```python
from build123d import *

# Parameters (mm, degrees)
BOSS_EXTRUDE1_DEPTH  = 4
MIRROR6_COPY_1_DEPTH = 4
MIRROR6_COPY_2_DEPTH = 4


with BuildPart() as part:
    # Sketch1 → Boss-Extrude1 (new body)
    with BuildSketch(Plane(origin=(0, 0, 0), x_dir=(1, 0, 0), z_dir=(0, 1, 0))):
        with BuildLine():
            Line((-290, 108.284271247), (-290, 0))
            Line((-290, 0), (-205.5, 0))
            ThreePointArc((-205.5, 0), (-202.131727984, 8.131727984), (-194, 11.5))
            Line((-194, 11.5), (-186, 11.5))
            ThreePointArc((-186, 11.5), (-177.868272016, 8.131727984), (-174.5, 0))
            Line((-174.5, 0), (0, 0))
            Line((0, 0), (0, 40))
            Line((0, 40), (-221.715728753, 40))
            Line((-221.715728753, 40), (-250, 68.284271247))
            Line((-250, 68.284271247), (-250, 108.284271247))
            Line((-250, 108.284271247), (-290, 108.284271247))
        make_face()
        with BuildLine():
            ThreePointArc((-207.499780644, 13.499780644), (-209.499780644, 15.499780644), (-207.499780644, 17.499780644))
            Line((-207.499780644, 17.499780644), (-203.499780644, 17.499780644))
            ThreePointArc((-203.499780644, 17.499780644), (-201.499780644, 15.499780644), (-203.499780644, 13.499780644))
            Line((-203.499780644, 13.499780644), (-207.499780644, 13.499780644))
        make_face(mode=Mode.SUBTRACT)
        with BuildLine():
            Line((-176.500219356, 17.499780644), (-172.500219356, 17.499780644))
            ThreePointArc((-172.500219356, 17.499780644), (-170.500219356, 15.499780644), (-172.500219356, 13.499780644))
            Line((-172.500219356, 13.499780644), (-176.500219356, 13.499780644))
            ThreePointArc((-176.500219356, 13.499780644), (-178.500219356, 15.499780644), (-176.500219356, 17.499780644))
        make_face(mode=Mode.SUBTRACT)
    boss_extrude1 = extrude(amount=BOSS_EXTRUDE1_DEPTH)

    # Mirror1: Boss-Extrude1 across plane
    add(boss_extrude1.mirror(Plane(origin=(0, 4, 0), x_dir=(1, 0, 0), z_dir=(0, 0, -1))))

    # Mirror5: Boss-Extrude1 across plane
    add(boss_extrude1.mirror(Plane(origin=(0, 4, 0), x_dir=(0, 0, 1), z_dir=(1, 0, 0))))

    # Mirror6 copy 1 sketch → Mirror6 copy 1 (add)
    with BuildSketch(Plane(origin=(0, 0, 0), x_dir=(-1, 0, 0), z_dir=(0, 1, 0))):
        with BuildLine():
            Line((-290, 108.284271247), (-290, 0))
            Line((-290, 0), (-205.5, 0))
            ThreePointArc((-205.5, 0), (-202.131727984, 8.131727984), (-194, 11.5))
            Line((-194, 11.5), (-186, 11.5))
            ThreePointArc((-186, 11.5), (-177.868272016, 8.131727984), (-174.5, 0))
            Line((-174.5, 0), (0, 0))
            Line((0, 0), (0, 40))
            Line((0, 40), (-221.715728753, 40))
            Line((-221.715728753, 40), (-250, 68.284271247))
            Line((-250, 68.284271247), (-250, 108.284271247))
            Line((-250, 108.284271247), (-290, 108.284271247))
        make_face()
        with BuildLine():
            ThreePointArc((-207.499780644, 13.499780644), (-209.499780644, 15.499780644), (-207.499780644, 17.499780644))
            Line((-207.499780644, 17.499780644), (-203.499780644, 17.499780644))
            ThreePointArc((-203.499780644, 17.499780644), (-201.499780644, 15.499780644), (-203.499780644, 13.499780644))
            Line((-203.499780644, 13.499780644), (-207.499780644, 13.499780644))
        make_face(mode=Mode.SUBTRACT)
        with BuildLine():
            Line((-176.500219356, 17.499780644), (-172.500219356, 17.499780644))
            ThreePointArc((-172.500219356, 17.499780644), (-170.500219356, 15.499780644), (-172.500219356, 13.499780644))
            Line((-172.500219356, 13.499780644), (-176.500219356, 13.499780644))
            ThreePointArc((-176.500219356, 13.499780644), (-178.500219356, 15.499780644), (-176.500219356, 17.499780644))
        make_face(mode=Mode.SUBTRACT)
    extrude(amount=MIRROR6_COPY_1_DEPTH)

    # Mirror6 copy 2 sketch → Mirror6 copy 2 (add)
    with BuildSketch(Plane(origin=(0, 0, 0), x_dir=(1, 0, 0), z_dir=(0, 1, 0))):
        with BuildLine():
            Line((-290, -108.284271247), (-290, 0))
            Line((-290, 0), (-205.5, 0))
            ThreePointArc((-205.5, 0), (-202.131727984, -8.131727984), (-194, -11.5))
            Line((-194, -11.5), (-186, -11.5))
            ThreePointArc((-186, -11.5), (-177.868272016, -8.131727984), (-174.5, 0))
            Line((-174.5, 0), (0, 0))
            Line((0, 0), (0, -40))
            Line((0, -40), (-221.715728753, -40))
            Line((-221.715728753, -40), (-250, -68.284271247))
            Line((-250, -68.284271247), (-250, -108.284271247))
            Line((-250, -108.284271247), (-290, -108.284271247))
        make_face()
        with BuildLine():
            ThreePointArc((-207.499780644, -13.499780644), (-209.499780644, -15.499780644), (-207.499780644, -17.499780644))
            Line((-207.499780644, -17.499780644), (-203.499780644, -17.499780644))
            ThreePointArc((-203.499780644, -17.499780644), (-201.499780644, -15.499780644), (-203.499780644, -13.499780644))
            Line((-203.499780644, -13.499780644), (-207.499780644, -13.499780644))
        make_face(mode=Mode.SUBTRACT)
        with BuildLine():
            Line((-176.500219356, -17.499780644), (-172.500219356, -17.499780644))
            ThreePointArc((-172.500219356, -17.499780644), (-170.500219356, -15.499780644), (-172.500219356, -13.499780644))
            Line((-172.500219356, -13.499780644), (-176.500219356, -13.499780644))
            ThreePointArc((-176.500219356, -13.499780644), (-178.500219356, -15.499780644), (-176.500219356, -17.499780644))
        make_face(mode=Mode.SUBTRACT)
    extrude(amount=MIRROR6_COPY_2_DEPTH)


solid = part.part
```
Model file for the job. Use its own axes, mm. A direction names the side the tool comes from. Give positions to 0.01 mm unless a question says otherwise; leave off trailing zeros. Loops run counter-clockwise (first coordinate to the right, second up) from the corner with the lowest first, then second, coordinate; pieces in that order, holes last. Notation, with made-up numbers: (-21.5, 85) -> (-2.5, 85) arc R15 cw to (-2.5, 105) -> close; hole circle Ø2 at (-27, 43.5). An arc over 180 degrees is marked (long way). Use CSV: the item, a comma, the result in double quotes. Start each with the question number.
1) Slice it at A-A on z = -84.5. Give the cut face in (x, y).
2) Flat gauge pins, fed straight in: pin 1 Ø2 at (x, y) = (174.5, 2.5) entering from +Z; pin 2 Ø1.2 at (x, y) = (103.5, 1) entering from -Z. Where does each tip first touch, or does it go through?
3) Mould opens along X. For faces 4 (the flat face through (4, 4, 2)), 5 (the flat face through (235.66, 1.972, -53.944)) say: released by +X, released by -X, zero draft, split by the parting line, or undercut.
4) Slice it at B-B on y = 0.9. Give the number of separate pieces and of enclosed holes in the cut face, plus the area to 3 significant figures.
5) Wall check: line 1 (X direction, y = 1.2, z = -15.5); line 2 (X direction, y = 1.35, z = -4); line 3 (X direction, y = 1.7, z = 99). Give the ranges that are in metal, low to high.
6) Tool access for faces 1 (the flat face through (4, 0, 2)), 2 (the flat face through (-235.66, 1.972, -53.944)), 3 (the flat face through (235.66, 1.972, 53.944)): list every direction of +Z, -Z, +X, -X, +Y, -Y with a clear straight run to the whole face (end or side of a thin tool).
7) Slice it at D-D on z = 45. Give the cut face in (x, y).
8) Slice it at C-C on x = 99. Give the cut face in (y, z), plus the area to 3 significant figures.
Computed values:
1,outline,"(-290, 0) -> (-250, 0) -> (-250, 4) -> (-290, 4) -> close; (250, 0) -> (290, 0) -> (290, 4) -> (250, 4) -> close"
2,pin 1,"stops at z = 40"
2,pin 2,"stops at z = -40"
3,face 4,"zero draft"
3,face 5,"undercut"
4,separate pieces,"1"
4,enclosed holes,"10"
4,area,"57,500 mm^2"
5,line 1,"x = -290 to -209.5, -201.5 to -178.5, -170.5 to 170.5, 178.5 to 201.5, 209.5 to 290"
5,line 2,"x = -290 to -204.78, -175.22 to 175.22, 204.78 to 290"
5,line 3,"x = -290 to -250, 250 to 290"
6,face 1,"+Z, -Z, +X, -X, -Y"
6,face 2,"-Z, +Y, -Y"
6,face 3,"+Z, +Y, -Y"
7,outline,"(-290, 0) -> (-226.72, 0) -> (-226.72, 4) -> (-290, 4) -> close; (226.72, 0) -> (290, 0) -> (290, 4) -> (226.72, 4) -> close"
8,outline,"(0, -40) -> (4, -40) -> (4, 40) -> (0, 40) -> close"
8,area,"320 mm^2"
